Build history of the part. All positions in model axes, mm. A direction names the side the tool comes from. Round coordinates to 2 decimals unless told otherwise and drop trailing zeros. Write each loop counter-clockwise with the first axis right and the second up, starting at its lowest first coordinate (ties: lowest second). Pieces come first, ordered by that corner, then holes. Notation, with made-up numbers: (36, 37) -> (91, 37) arc R19 cw to (91, 52) -> close; hole circle Ø6 at (83, -15.75). An arc over 180 degrees is marked (long way). Answer in a Markdown table with one row per item.
```python
from build123d import *

# Parameters (mm, degrees)
BOSS_EXTRUDE1_DEPTH = 2070.1
SKETCH2_R           = 6.35
CUT_EXTRUDE1_DEPTH  = 2073.54194621
SKETCH3_R           = 3.274297192
CUT_EXTRUDE2_DEPTH  = 2073.54194621
CUT_EXTRUDE3_REACH  = 2074.542
SKETCH4_R           = 1.905
CUT_EXTRUDE4_DEPTH  = 1917.7


with BuildPart() as part:
    # Sketch1 → Boss-Extrude1 (new body)
    with BuildSketch(Plane.XY):
        with BuildLine():
            Line((6.35, 0), (64.77, 0))
            ThreePointArc((64.77, 0), (69.260128061, 1.859871939), (71.12, 6.35))
            Line((71.12, 6.35), (71.12, 64.77))
            ThreePointArc((71.12, 64.77), (69.260128061, 69.260128061), (64.77, 71.12))
            Line((64.77, 71.12), (6.35, 71.12))
            ThreePointArc((6.35, 71.12), (1.859871939, 69.260128061), (0, 64.77))
            Line((0, 64.77), (0, 6.35))
            ThreePointArc((0, 6.35), (1.859871939, 1.859871939), (6.35, 0))
        make_face()
        with BuildLine():
            Line((6.35, 3.175), (64.77, 3.175))
            ThreePointArc((64.77, 3.175), (67.01506403, 4.10493597), (67.945, 6.35))
            Line((67.945, 6.35), (67.945, 64.77))
            ThreePointArc((67.945, 64.77), (67.01506403, 67.01506403), (64.77, 67.945))
            Line((64.77, 67.945), (6.35, 67.945))
            ThreePointArc((6.35, 67.945), (4.10493597, 67.01506403), (3.175, 64.77))
            Line((3.175, 64.77), (3.175, 6.35))
            ThreePointArc((3.175, 6.35), (4.10493597, 4.10493597), (6.35, 3.175))
        make_face(mode=Mode.SUBTRACT)
    extrude(amount=BOSS_EXTRUDE1_DEPTH)

    # Sketch2 → Cut-Extrude1 (cut, through all)
    with BuildSketch(Plane(origin=(0, 0, 0), x_dir=(1, 0, 0), z_dir=(0, 1, 0))):
        with Locations(Location((35.56, -101.6, 0), (0, 0, 90))):
            Circle(SKETCH2_R)
        with Locations(Location((35.56, -279.4, 0), (0, 0, 90))):
            Circle(SKETCH2_R)
    extrude(amount=CUT_EXTRUDE1_DEPTH, mode=Mode.SUBTRACT)

    # Sketch3 → Cut-Extrude2 (cut, through all)
    with BuildSketch(Plane.ZY):
        with Locations((12.7, 53.975)):
            Circle(SKETCH3_R)
        with Locations((12.7, 17.145)):
            Circle(SKETCH3_R)
        with Locations((63.5, 17.145)):
            Circle(SKETCH3_R)
        with Locations((63.5, 53.975)):
            Circle(SKETCH3_R)
    extrude(amount=-CUT_EXTRUDE2_DEPTH, mode=Mode.SUBTRACT)

    # Sketch4 → Cut-Extrude3 (cut, up to next)
    with BuildSketch(Plane(origin=(0, 71.12, 0), x_dir=(1, 0, 0), z_dir=(0, 1, 0)), mode=Mode.PRIVATE) as cut_extrude3_sk1:
        with Locations(Location((13.335, -1508.125, 0), (0, 0, 270))):
            Circle(SKETCH4_R)
    cut_extrude3_tool1 = extrude(cut_extrude3_sk1.sketch, amount=-CUT_EXTRUDE3_REACH, mode=Mode.PRIVATE) & part.part
    # Sketch4 → Cut-Extrude3 (cut, up to next)
    with BuildSketch(Plane(origin=(0, 71.12, 0), x_dir=(1, 0, 0), z_dir=(0, 1, 0)), mode=Mode.PRIVATE) as cut_extrude3_sk2:
        with Locations(Location((57.785, -1508.125, 0), (0, 0, 270))):
            Circle(SKETCH4_R)
    cut_extrude3_tool2 = extrude(cut_extrude3_sk2.sketch, amount=-CUT_EXTRUDE3_REACH, mode=Mode.PRIVATE) & part.part
    # Sketch4 → Cut-Extrude3 (cut, up to next)
    with BuildSketch(Plane(origin=(0, 71.12, 0), x_dir=(1, 0, 0), z_dir=(0, 1, 0)), mode=Mode.PRIVATE) as cut_extrude3_sk3:
        with Locations(Location((57.785, -1565.275, 0), (0, 0, 270))):
            Circle(SKETCH4_R)
    cut_extrude3_tool3 = extrude(cut_extrude3_sk3.sketch, amount=-CUT_EXTRUDE3_REACH, mode=Mode.PRIVATE) & part.part
    # Sketch4 → Cut-Extrude3 (cut, up to next)
    with BuildSketch(Plane(origin=(0, 71.12, 0), x_dir=(1, 0, 0), z_dir=(0, 1, 0)), mode=Mode.PRIVATE) as cut_extrude3_sk4:
        with Locations(Location((13.335, -1565.275, 0), (0, 0, 270))):
            Circle(SKETCH4_R)
    cut_extrude3_tool4 = extrude(cut_extrude3_sk4.sketch, amount=-CUT_EXTRUDE3_REACH, mode=Mode.PRIVATE) & part.part
    # Sketch4 → Cut-Extrude3 (cut, up to next)
    with BuildSketch(Plane(origin=(0, 71.12, 0), x_dir=(1, 0, 0), z_dir=(0, 1, 0)), mode=Mode.PRIVATE) as cut_extrude3_sk5:
        with Locations(Location((13.335, -1133.475, 0), (0, 0, 270))):
            Circle(SKETCH4_R)
    cut_extrude3_tool5 = extrude(cut_extrude3_sk5.sketch, amount=-CUT_EXTRUDE3_REACH, mode=Mode.PRIVATE) & part.part
    # Sketch4 → Cut-Extrude3 (cut, up to next)
    with BuildSketch(Plane(origin=(0, 71.12, 0), x_dir=(1, 0, 0), z_dir=(0, 1, 0)), mode=Mode.PRIVATE) as cut_extrude3_sk6:
        with Locations(Location((57.785, -1133.475, 0), (0, 0, 270))):
            Circle(SKETCH4_R)
    cut_extrude3_tool6 = extrude(cut_extrude3_sk6.sketch, amount=-CUT_EXTRUDE3_REACH, mode=Mode.PRIVATE) & part.part
    # Sketch4 → Cut-Extrude3 (cut, up to next)
    with BuildSketch(Plane(origin=(0, 71.12, 0), x_dir=(1, 0, 0), z_dir=(0, 1, 0)), mode=Mode.PRIVATE) as cut_extrude3_sk7:
        with Locations(Location((57.785, -1190.625, 0), (0, 0, 270))):
            Circle(SKETCH4_R)
    cut_extrude3_tool7 = extrude(cut_extrude3_sk7.sketch, amount=-CUT_EXTRUDE3_REACH, mode=Mode.PRIVATE) & part.part
    # Sketch4 → Cut-Extrude3 (cut, up to next)
    with BuildSketch(Plane(origin=(0, 71.12, 0), x_dir=(1, 0, 0), z_dir=(0, 1, 0)), mode=Mode.PRIVATE) as cut_extrude3_sk8:
        with Locations(Location((13.335, -1190.625, 0), (0, 0, 270))):
            Circle(SKETCH4_R)
    cut_extrude3_tool8 = extrude(cut_extrude3_sk8.sketch, amount=-CUT_EXTRUDE3_REACH, mode=Mode.PRIVATE) & part.part
    add(cut_extrude3_tool1.solids().sort_by_distance((13.335, 71.12, 1508.125))[0], mode=Mode.SUBTRACT)
    add(cut_extrude3_tool2.solids().sort_by_distance((57.785, 71.12, 1508.125))[0], mode=Mode.SUBTRACT)
    add(cut_extrude3_tool3.solids().sort_by_distance((57.785, 71.12, 1565.275))[0], mode=Mode.SUBTRACT)
    add(cut_extrude3_tool4.solids().sort_by_distance((13.335, 71.12, 1565.275))[0], mode=Mode.SUBTRACT)
    add(cut_extrude3_tool5.solids().sort_by_distance((13.335, 71.12, 1133.475))[0], mode=Mode.SUBTRACT)
    add(cut_extrude3_tool6.solids().sort_by_distance((57.785, 71.12, 1133.475))[0], mode=Mode.SUBTRACT)
    add(cut_extrude3_tool7.solids().sort_by_distance((57.785, 71.12, 1190.625))[0], mode=Mode.SUBTRACT)
    add(cut_extrude3_tool8.solids().sort_by_distance((13.335, 71.12, 1190.625))[0], mode=Mode.SUBTRACT)

    # Sketch5 → Cut-Extrude4 (cut)
    with BuildSketch(Plane(origin=(0, 0, 0), x_dir=(-1, 0, 0), z_dir=(0, 0, -1))):
        with BuildLine():
            Line((0, 6.35), (0, 64.77))
            ThreePointArc((0, 64.77), (-1.859871939, 69.260128061), (-6.35, 71.12))
            Line((-6.35, 71.12), (-64.77, 71.12))
            ThreePointArc((-64.77, 71.12), (-69.260128061, 69.260128061), (-71.12, 64.77))
            Line((-71.12, 64.77), (-71.12, 6.35))
            ThreePointArc((-71.12, 6.35), (-69.260128061, 1.859871939), (-64.77, 0))
            Line((-64.77, 0), (-6.35, 0))
            ThreePointArc((-6.35, 0), (-1.859871939, 1.859871939), (0, 6.35))
        make_face()
    extrude(amount=-CUT_EXTRUDE4_DEPTH, mode=Mode.SUBTRACT)


solid = part.part
```
Q1. Saw through at A-A on x = 32. Write the cut outline in (y, z) (3 decimals).
A:
| item | result |
|---|---|
| outline | (0, 1917.7) -> (3.175, 1917.7) -> (3.175, 2070.1) -> (0, 2070.1) -> close; (67.945, 1917.7) -> (71.12, 1917.7) -> (71.12, 2070.1) -> (67.945, 2070.1) -> close |
Q2. Saw through at C-C on z = 2001. Write the cut outline in (x, y) (3 decimals).
A:
| item | result |
|---|---|
| outline | (0, 6.35) arc R6.35 ccw to (6.35, 0) -> (64.77, 0) arc R6.35 ccw to (71.12, 6.35) -> (71.12, 64.77) arc R6.35 ccw to (64.77, 71.12) -> (6.35, 71.12) arc R6.35 ccw to (0, 64.77) -> close; hole (3.175, 6.35) arc R3.175 ccw to (6.35, 3.175) -> (64.77, 3.175) arc R3.175 ccw to (67.945, 6.35) -> (67.945, 64.77) arc R3.175 ccw to (64.77, 67.945) -> (6.35, 67.945) arc R3.175 ccw to (3.175, 64.77) -> close |
Q3. Wall check: line 1 (Y direction, x = 38, z = 2062) (3 decimals); line 2 (Y direction, x = 67.5, z = 1937). Give the ranges that are in metal, low to high. Write a range as [from, to].
A:
| item | result |
|---|---|
| line 1 | [0, 3.175], [67.945, 71.12] |
| line 2 | [0.62, 4.73], [66.39, 70.5] |
Q4. Two-plate mould, pull along Y, no slides. Class faces 3 (the flat face through (1, 36, 2070.1)), 4 (the cylindrical face through (4.08, 4.13, 1992.83)), 5 (the cylindrical face through (67.04, 66.99, 1992.83)), 6 (the flat face through (36, 71.12, 1993)): released by +Y, released by -Y, zero draft, split by the parting line, or undercut.
A:
| item | result |
|---|---|
| face 3 | zero draft |
| face 4 | undercut |
| face 5 | undercut |
| face 6 | released by +Y |
Q5. Which spindle directions (+Z, -Z, +X, -X, +Y, -Y) get a long thin tool onto all of the face, cutting with end or side? Do faces 1 (the flat face through (67.945, 35, 1993)), 2 (the flat face through (70, 36, 1917.7)). Say none if no direction does.
A:
| item | result |
|---|---|
| face 1 | +Z, -Z |
| face 2 | -Z, +X, -X, +Y, -Y |
